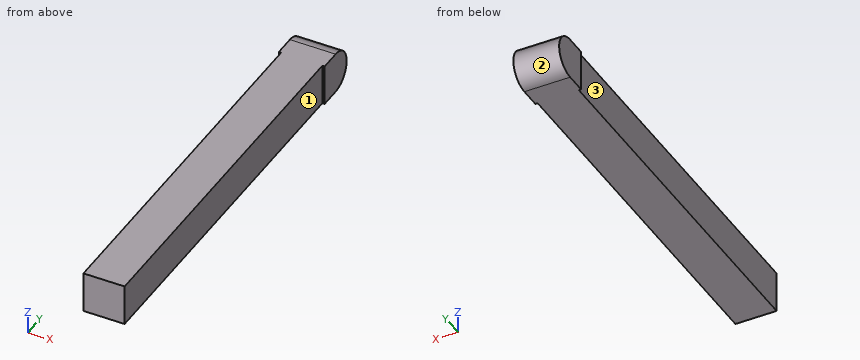
from build123d import *

# Parameters (mm, degrees)
SKETCH_1_W          = 18
SKETCH_1_H          = 18
EXTRUDE_1_DEPTH     = 160
SKETCH_2_W          = 18
SKETCH_2_H          = 18
EXTRUDE_2_DEPTH     = 2
SKETCH_3_W          = 20
SKETCH_3_H          = 18
EXTRUDE_4_DEPTH     = 18
CUT_EXTRUDE_1_DEPTH = 21


with BuildPart() as part:
    # 草图1 → 凸台-拉伸1 (new body)
    with BuildSketch(Plane(origin=(0, 0, 0), x_dir=(1, 0, 0), z_dir=(0, 1, 0))):
        Rectangle(SKETCH_1_W, SKETCH_1_H)
    extrude(amount=EXTRUDE_1_DEPTH)

    # 草图2 → 凸台-拉伸2 (add)
    with BuildSketch(Plane(origin=(0, 160, 0), x_dir=(1, 0, 0), z_dir=(0, 1, 0))):
        Rectangle(SKETCH_2_W, SKETCH_2_H)
    extrude(amount=EXTRUDE_2_DEPTH)

    # 草图3 → 凸台-拉伸4 (add)
    with BuildSketch(Plane(origin=(0, 162, 0), x_dir=(1, 0, 0), z_dir=(0, 1, 0))):
        Rectangle(SKETCH_3_W, SKETCH_3_H)
    extrude(amount=EXTRUDE_4_DEPTH)

    # 草图4 → 切除-拉伸1 (cut, through all)
    with BuildSketch(Plane.ZY.offset(10)):
        with BuildLine():
            Line((-9, 171), (-9, 185))
            Line((-9, 185), (9, 185))
            Line((9, 185), (9, 171))
            ThreePointArc((9, 171), (0, 180), (-9, 171))
        make_face()
    extrude(amount=-CUT_EXTRUDE_1_DEPTH, mode=Mode.SUBTRACT)


solid = part.part
The model under review builds one solid part; all positions refer to its coordinate system, in mm. Face numbers are marked on the shaded views. A direction names the side the tool comes from. Round coordinates to 2 decimals unless told otherwise and drop trailing zeros. Write each loop counter-clockwise with the first axis right and the second up, starting at its lowest first coordinate (ties: lowest second). Pieces come first, ordered by that corner, then holes. Notation, with made-up numbers: (-24, 21) - (-18, 21) arc R24 ccw to (-18, 49) - close; hole circle Ø3 at (-28, -13). An arc over 180 degrees is marked (long way). One line per item, written item: value. Start each with the question number.
1. Consider section C-C on z = 7. Write out the cut boundary in (x, y).
2. To check wall thickness, follow L1, parallel to X at y = 116.5, z = 2.75; L2, parallel to Y at x = -7, z = 0; L3, parallel to Z at x = 2.5, y = 171.5. State the ranges of each line that lie inside material, in increasing order. Write a range as from..to.
3. Machinability: for the marked faces 1, 2 and 3, which of the approach directions +Z, -Z, +X, -X, +Y, -Y give a long, thin tool a straight path to every point of the face, cutting with its end or side? Answer none if there is none.
4. Consider section B-B on y = 116. Write out the cut boundary in (x, z).
5. Consider section A-A on z = 0. Write out the cut boundary in (x, y).
6. Clearance check with flat-ended pins moving along their axes: P1, Ø3, axis at y = 113, z = -1.5, coming from the +X side; P2, Ø10, axis at y = 143, z = 2.5, coming from the -X side; P3, Ø0.8, axis at x = -9.5, z = 2, coming from the -Y side. State where each tip first meets the part, or that it passes through.
Checks:
1. outline: (-10, 162) - (-9, 162) - (-9, 0) - (9, 0) - (9, 162) - (10, 162) - (10, 176.66) - (-10, 176.66) - close
2. L1: x = -9..9
2. L2: y = 0..180
2. L3: z = -8.99..8.99
3. face 1: +Z, -Z, +X, -Y
3. face 2: +X, -X, +Y
3. face 3: +Z, -Z, -X, -Y
4. outline: (-9, -9) - (9, -9) - (9, 9) - (-9, 9) - close
5. outline: (-10, 162) - (-9, 162) - (-9, 0) - (9, 0) - (9, 162) - (10, 162) - (10, 180) - (-10, 180) - close
6. P1: stops at x = 9
6. P2: stops at x = -9
6. P3: stops at y = 162
